from build123d import *

# Parameters (mm, degrees)
F1_DEPTH = 22.225
F2_DEPTH = 50.8
F3_DEPTH = 38.1


with BuildPart() as f1:
    # F0 (on Top) → F1 (new body)
    with BuildSketch(Plane.XY):
        with BuildLine():
            ThreePointArc((4.5574981074, -34.6263604209), (25.9122606637, -23.4160281067), (34.9095515761, -1.0386692217))
            Line((34.9095515761, -1.0386692217), (22.2151691848, -0.6609713229))
            ThreePointArc((22.2151691848, -0.6609713229), (15.2411194712, -16.1758740804), (-0.6609713229, -22.2151691848))
            Line((-0.6609713229, -22.2151691848), (-1.0386692217, -34.9095515761))
            ThreePointArc((-1.0386692217, -34.9095515761), (-0.5193920499, -34.9211376805), (0, -34.925))
            Line((0, -34.925), (4.5574981074, -34.6263604209))
        make_face()
        with BuildLine():
            ThreePointArc((34.9095515761, -1.0386692217), (34.9211376805, -0.5193920499), (34.925, 0))
            ThreePointArc((34.925, 0), (27.5419497881, 21.4754889786), (8.514312706, 33.871257788))
            Line((8.514312706, 33.871257788), (0, 34.925))
            ThreePointArc((0, 34.925), (-34.9211376805, 0.5193920499), (-1.0386692217, -34.9095515761))
            Line((-1.0386692217, -34.9095515761), (-0.6609713229, -22.2151691848))
            ThreePointArc((-0.6609713229, -22.2151691848), (-15.4799957582, 15.9474247553), (22.225, 0))
            ThreePointArc((22.225, 0), (22.2225421603, -0.3305222136), (22.2151691848, -0.6609713229))
            Line((22.2151691848, -0.6609713229), (34.9095515761, -1.0386692217))
        make_face()
        with BuildLine():
            Line((111.0758459241, -3.3048566146), (34.9095515761, -1.0386692217))
            ThreePointArc((34.9095515761, -1.0386692217), (25.9122606637, -23.4160281067), (4.5574981074, -34.6263604209))
            Line((4.5574981074, -34.6263604209), (133.2910151089, -26.1908279375))
            ThreePointArc((133.2910151089, -26.1908279375), (117.3435903536, -19.4458236957), (111.0758459241, -3.3048566146))
        make_face()
        with BuildLine():
            ThreePointArc((8.514312706, 33.871257788), (27.5419497881, 21.4754889786), (34.925, 0))
            ThreePointArc((34.925, 0), (34.9211376805, -0.5193920499), (34.9095515761, -1.0386692217))
            Line((34.9095515761, -1.0386692217), (111.0758459241, -3.3048566146))
            ThreePointArc((111.0758459241, -3.3048566146), (117.8110193507, 11.9815968178), (133.2910151089, 18.2591720625))
            Line((133.2910151089, 18.2591720625), (133.2910151089, 18.4287337781))
            Line((133.2910151089, 18.4287337781), (8.514312706, 33.871257788))
        make_face()
        with BuildLine():
            ThreePointArc((133.2910151089, 18.2591720625), (117.8110193507, 11.9815968178), (111.0758459241, -3.3048566146))
            ThreePointArc((111.0758459241, -3.3048566146), (117.3435903536, -19.4458236957), (133.2910151089, -26.1908279375))
            ThreePointArc((133.2910151089, -26.1908279375), (149.0064633208, -19.6812761494), (155.5160151089, -3.9658279375))
            ThreePointArc((155.5160151089, -3.9658279375), (149.0064633208, 11.7496202744), (133.2910151089, 18.2591720625))
        make_face()
        with BuildLine():
            ThreePointArc((145.9910151089, -3.9658279375), (133.1021452726, -16.6644234577), (120.5966327176, -3.5881300387))
            ThreePointArc((120.5966327176, -3.5881300387), (133.4798849453, 8.7327675827), (145.9910151089, -3.9658279375))
        make_face(mode=Mode.SUBTRACT)
    extrude(amount=F1_DEPTH)

    # F0 (on Top) → F2 (join)
    with BuildSketch(Plane.XY):
        with BuildLine():
            ThreePointArc((4.5574981074, -34.6263604209), (25.9122606637, -23.4160281067), (34.9095515761, -1.0386692217))
            Line((34.9095515761, -1.0386692217), (22.2151691848, -0.6609713229))
            ThreePointArc((22.2151691848, -0.6609713229), (15.2411194712, -16.1758740804), (-0.6609713229, -22.2151691848))
            Line((-0.6609713229, -22.2151691848), (-1.0386692217, -34.9095515761))
            ThreePointArc((-1.0386692217, -34.9095515761), (-0.5193920499, -34.9211376805), (0, -34.925))
            Line((0, -34.925), (4.5574981074, -34.6263604209))
        make_face()
        with BuildLine():
            ThreePointArc((34.9095515761, -1.0386692217), (34.9211376805, -0.5193920499), (34.925, 0))
            ThreePointArc((34.925, 0), (27.5419497881, 21.4754889786), (8.514312706, 33.871257788))
            Line((8.514312706, 33.871257788), (0, 34.925))
            ThreePointArc((0, 34.925), (-34.9211376805, 0.5193920499), (-1.0386692217, -34.9095515761))
            Line((-1.0386692217, -34.9095515761), (-0.6609713229, -22.2151691848))
            ThreePointArc((-0.6609713229, -22.2151691848), (-15.4799957582, 15.9474247553), (22.225, 0))
            ThreePointArc((22.225, 0), (22.2225421603, -0.3305222136), (22.2151691848, -0.6609713229))
            Line((22.2151691848, -0.6609713229), (34.9095515761, -1.0386692217))
        make_face()
    extrude(amount=F2_DEPTH)

    # F0 (on Top) → F3 (join)
    with BuildSketch(Plane.XY):
        with BuildLine():
            ThreePointArc((133.2910151089, 18.2591720625), (117.8110193507, 11.9815968178), (111.0758459241, -3.3048566146))
            ThreePointArc((111.0758459241, -3.3048566146), (117.3435903536, -19.4458236957), (133.2910151089, -26.1908279375))
            ThreePointArc((133.2910151089, -26.1908279375), (149.0064633208, -19.6812761494), (155.5160151089, -3.9658279375))
            ThreePointArc((155.5160151089, -3.9658279375), (149.0064633208, 11.7496202744), (133.2910151089, 18.2591720625))
        make_face()
        with BuildLine():
            ThreePointArc((145.9910151089, -3.9658279375), (133.1021452726, -16.6644234577), (120.5966327176, -3.5881300387))
            ThreePointArc((120.5966327176, -3.5881300387), (133.4798849453, 8.7327675827), (145.9910151089, -3.9658279375))
        make_face(mode=Mode.SUBTRACT)
    extrude(amount=F3_DEPTH)


solid = f1.part
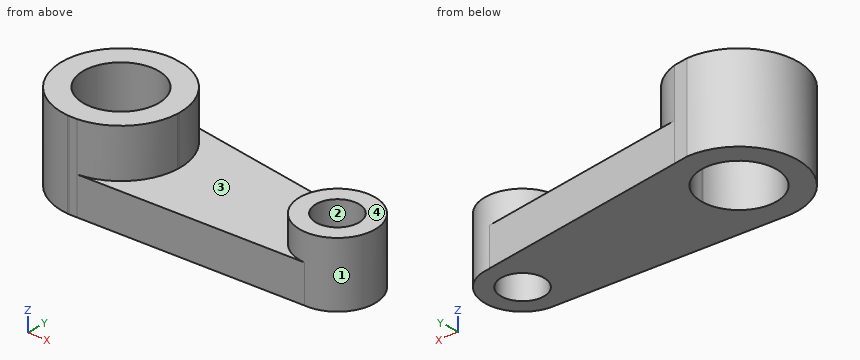
Build history of the part. All positions in model axes, mm. Face numbers are marked on the shaded views. A direction names the side the tool comes from. Coordinates: 2 decimals unless noted, no trailing zeros. Write each loop counter-clockwise with the first axis right and the second up, starting at its lowest first coordinate (ties: lowest second). Pieces come first, ordered by that corner, then holes.
(1) Cut at A-A on y = 16.5. List the corners of the cut face in (x, z) (3 decimals), and give its area (3 significant figures).
(2) 3-axis set-ups, long thin cutter, end or side, ignore diameter. For the marked faces 1 and 2: which of +Z, -Z, +X, -X, +Y, -Y reach the whole face in a straight line?
(3) Mould opens along X. For the marked faces 3 and 4 say: pulls with the +X half, pulls with the -X half, needs draft (parallel to the pull), parting line crosses it, or undercut.
(4) Pin check, flat tips, straight feed: pin 1 Ø1.5 at (x, y) = (63.5, -18.5) entering from +Z (3 decimals); pin 2 Ø1.5 at (y, z) = (18, 13.5) entering from -X; pin 3 Ø8 at (x, z) = (58.5, 14) entering from -Y. Stop position of each tip, or through.
(5) Cut at D-D on y = 4. List the corners of the cut face in (x, z) (3 decimals), and give its area (3 significant figures).
(6) Cut at C-C on x = 17.5. List the corners of the cut face in (y, z) (3 decimals).
(7) Drill centre lines: line 1 (Y direction, x = 0, z = 22.5) (3 decimals); line 2 (X direction, y = -12, z = 18.5); line 3 (X direction, y = -3.5, z = 22). Where is each one in solid material? Low to high.
Working result:
1. outline: (-30.782, 0) - (-14.89, 0) - (-14.89, 50.8) - (-30.782, 50.8) - close; (14.89, 0) - (141.957, 0) - (141.957, 38.1) - (124.625, 38.1) - (124.625, 22.225) - (30.782, 22.225) - (30.782, 50.8) - (14.89, 50.8) - close
1. area: 4,360 mm2
2. face 1: +Z
2. face 2: +Z, -Z
3. face 3: undercut
3. face 4: needs draft
4. pin 1: stops at z = 22.225
4. pin 2: stops at x = -30.37
4. pin 3: stops at y = -31.35
5. outline: (-34.695, 0) - (-21.862, 0) - (-21.862, 50.8) - (-34.695, 50.8) - close; (21.862, 0) - (123.4, 0) - (123.4, 38.1) - (112.543, 38.1) - (112.543, 22.225) - (34.695, 22.225) - (34.695, 50.8) - (21.862, 50.8) - close; (143.182, 0) - (154.039, 0) - (154.039, 38.1) - (143.182, 38.1) - close
5. area: 3,860 mm2
6. outline: (-33.778, 0) - (-13.7, 0) - (-13.7, 50.8) - (-30.224, 50.8) - (-30.224, 22.225) - (-33.778, 22.225) - close; (13.7, 0) - (32.759, 0) - (32.759, 22.225) - (30.224, 22.225) - (30.224, 50.8) - (13.7, 50.8) - close
7. line 1: y = -34.925 to -22.225, 22.225 to 34.925
7. line 2: x = -32.8 to -18.71, 18.71 to 123.46, 143.13 to 154.01
7. line 3: x = -34.75 to -21.95, 21.95 to 120.6, 145.98 to 155.51
